CAD build for the part. Positions are in the model's coordinates, mm. Face numbers are marked on the shaded views. A direction names the side the tool comes from. Give positions to 0.01 mm unless a question says otherwise; leave off trailing zeros. Order: outer loops, then holes, each group sorted by start corner. A loop starts at its lowest first (then second) coordinate and runs counter-clockwise, first axis right, second up. Notation, with made-up numbers: (75, -37) -> (100, -37) arc R31 ccw to (100, 1) -> close; hole circle Ø2 at (67, 25.25). An arc over 180 degrees is marked (long way). Answer as CSV lines item,"result".
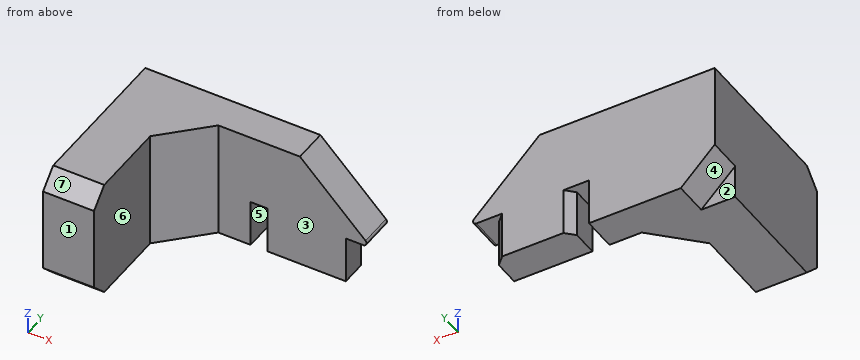
```python
from build123d import *

# Parameters (mm, degrees)
BOSS_EXTRUDE1_DEPTH = 17.78
SKETCH4_W           = 2.54
SKETCH4_H           = 7.112
CUT_EXTRUDE2_DEPTH  = 6.08
CUT_EXTRUDE1_DEPTH  = 5.08
CHAMFER3_SIZE       = 2.54
FILLET2_R           = 0.508
CHAMFER4_SIZE       = 1.27


with BuildPart() as part:
    # Sketch1 → Boss-Extrude1 (new body)
    with BuildSketch(Plane.XY):
        Polygon((0, 0), (0, 25.4), (43.18, 25.4), (43.18, 20.32), (13.97, 20.32), (7.62, 13.97), (7.62, 0), align=None)
    extrude(amount=BOSS_EXTRUDE1_DEPTH)

    # Sketch4 → Cut-Extrude2 (cut, through all)
    with BuildSketch(Plane.XZ.offset(-20.32)):
        with Locations((20.066, 3.556)):
            Rectangle(SKETCH4_W, SKETCH4_H)
        Polygon((33.02, 0), (33.02, 7.112), (36.83, 7.112), (26.162, 17.78), (43.18, 17.78), (43.18, 0), align=None)
    extrude(amount=-CUT_EXTRUDE2_DEPTH, mode=Mode.SUBTRACT)

    # Sketch3 → Cut-Extrude1 (cut)
    with BuildSketch(Plane(origin=(0, 25.4, 0), x_dir=(1, 0, 0), z_dir=(0, 1, 0))):
        Polygon((0, 0), (0, -5.08), (5.08, 0), align=None)
    extrude(amount=-CUT_EXTRUDE1_DEPTH, mode=Mode.SUBTRACT)

    # Chamfer3
    chamfer3_edges = [part.edges().sort_by_distance(p)[0] for p in [
        (3.81, 0, 0),
        (3.81, 0, 17.78),
    ]]
    chamfer(chamfer3_edges, length=CHAMFER3_SIZE)

    # Fillet2
    fillet2_edges = [part.edges().sort_by_distance(p)[0] for p in [
        (36.83, 22.86, 7.112),
    ]]
    fillet(fillet2_edges, radius=FILLET2_R)

    # Chamfer4
    chamfer4_edges = [part.edges().sort_by_distance(p)[0] for p in [
        (21.336, 25.4, 3.556),
        (33.02, 25.4, 3.556),
    ]]
    chamfer(chamfer4_edges, length=CHAMFER4_SIZE)


solid = part.part
```
1) Pull direction X, two halves, no side cores. Call the marked faces 4, 5, 6 and 7: pulls with the +X half, pulls with the -X half, needs draft (parallel to the pull), parting line crosses it, or undercut.
Data:
face 4,"pulls with the -X half"
face 5,"undercut"
face 6,"pulls with the +X half"
face 7,"needs draft"
2) Band-saw the part on C-C, the plane z = 9. Write the cut outline in (x, y), then the cut area to 3 significant figures.
Data:
outline,"(0, 0) -> (7.62, 0) -> (7.62, 13.97) -> (13.97, 20.32) -> (34.94, 20.32) -> (34.94, 25.4) -> (0, 25.4) -> close"
area,"353 mm2"
3) Which spindle directions (+Z, -Z, +X, -X, +Y, -Y) get a long thin tool onto all of the face, cutting with end or side? Do the marked faces 1, 2 and 3. Say none if no direction does.
Data:
face 1,"+Z, -Z, +X, -X, -Y"
face 2,"-Z, -X, +Y"
face 3,"+Z, -Z, +X, -Y"
4) Band-saw the part on D-D, the plane y = 6. Write the cut outline in (x, z).
Data:
outline,"(0, 0) -> (7.62, 0) -> (7.62, 17.78) -> (0, 17.78) -> close"
5) Wall check: line 1 along X through (y, z) = (8.5, 10.75); line 2 along Y through (x, z) = (26, 1.75); line 3 along X through (y, z) = (19, 13.5). Give the ranges that are in metal, low to high. Write a range as [from, to].
Data:
line 1,"x = [0, 7.62]"
line 2,"y = [20.32, 25.4]"
line 3,"x = [0, 12.65]"
6) Pin check, flat tips, straight feed: P1, Ø8, axis at x = 20, z = 15.5, coming from the -Y side; P2, Ø5, axis at y = 12.5, z = 5, coming from the +X side; P3, Ø4, axis at y = 22.5, z = 2.5, coming from the +X side. Stop position of each tip, or through.
Data:
P1,"stops at y = 20.32"
P2,"stops at x = 8.65"
P3,"stops at x = 33.02"
7) Band-saw the part on B-B, the plane z = 5.75. Write the cut outline in (x, y).
Data:
outline,"(0, 0) -> (7.62, 0) -> (7.62, 13.97) -> (13.97, 20.32) -> (18.8, 20.32) -> (18.8, 25.4) -> (0, 25.4) -> close; (21.34, 20.32) -> (33.02, 20.32) -> (33.02, 24.13) -> (31.75, 25.4) -> (22.61, 25.4) -> (21.34, 24.13) -> close"
8) Band-saw the part on A-A, the plane z = 3. Write the cut outline in (x, y), then the cut area to 3 significant figures.
Data:
outline,"(0, 0) -> (7.62, 0) -> (7.62, 13.97) -> (13.97, 20.32) -> (18.8, 20.32) -> (18.8, 25.4) -> (2.08, 25.4) -> (2.08, 20.32) -> (0, 20.32) -> close; (21.34, 20.32) -> (33.02, 20.32) -> (33.02, 24.13) -> (31.75, 25.4) -> (22.61, 25.4) -> (21.34, 24.13) -> close"
area,"318 mm2"
